The listing builds one solid part. Answer for the finished solid, in the listing's coordinates (mm). Face numbers are marked on the shaded views. A direction names the side the tool comes from. Coordinates: 2 decimals unless noted, no trailing zeros. Write each loop counter-clockwise with the first axis right and the second up, starting at its lowest first coordinate (ties: lowest second). Pieces come first, ordered by that corner, then holes.
(1) The part is cut by section A-A on z = 0. Determine the outline of the cut face in (x, y), plus the area to 3 significant figures.
(2) Given P1, Ø1.5, axis at y = 50.5, z = -0.5, coming from the +X side; P2, Ø18, axis at x = 49, z = -6.5, coming from the +Y side, each flat-ended and moving along its own axis, determine where each tip first touches the part or whether it passes through.
(3) Which of the six approach directions +Z, -Z, +X, -X, +Y, -Y give full straight-line access (tool end or side, diameter ignored) to the marked faces 1 and 2?
(4) The part is cut by section B-B on y = 60. Determine the outline of the cut face in (x, z), plus the area to 3 significant figures.
(5) The part is cut by section D-D on z = -5.5. Determine the outline of the cut face in (x, y).
(6) Straight lines are drawn through the part: line 1 (Z direction, x = 4, y = 20); line 2 (Y direction, x = 3.8, z = 0); line 3 (Y direction, x = 4.55, z = 0). For each, find the intervals that lie inside material, in ascending order.
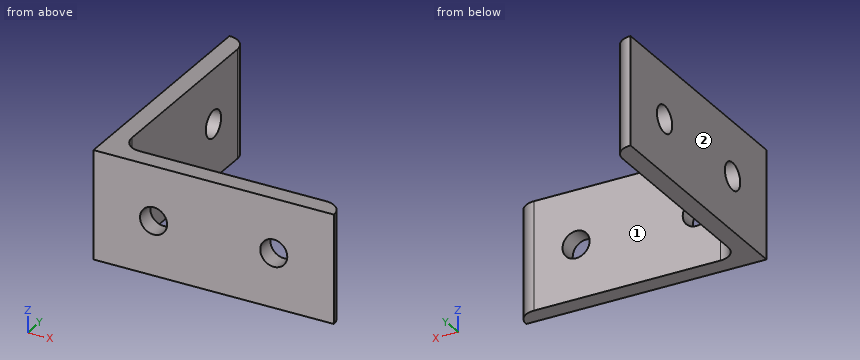
from build123d import *

# Parameters (mm, degrees)
BOSS_EXTRUDE1_DEPTH = 18
SKETCH2_R           = 4.5
CUT_EXTRUDE1_DEPTH  = 81
SKETCH3_R           = 4.5
CUT_EXTRUDE2_DEPTH  = 81


with BuildPart() as part:
    # Sketch1 → Boss-Extrude1 (new body, symmetric)
    with BuildSketch(Plane.XY):
        with BuildLine():
            Line((0, 0), (0, 80))
            ThreePointArc((0, 80), (4.242640687, 78.242640687), (6, 74))
            Line((6, 74), (6, 12))
            ThreePointArc((6, 12), (7.757359313, 7.757359313), (12, 6))
            Line((12, 6), (74, 6))
            ThreePointArc((74, 6), (78.242640687, 4.242640687), (80, 0))
            Line((80, 0), (0, 0))
        make_face()
    extrude(amount=BOSS_EXTRUDE1_DEPTH, both=True)

    # Sketch2 → Cut-Extrude1 (cut, through all)
    with BuildSketch(Plane(origin=(0, 0, 0), x_dir=(1, 0, 0), z_dir=(0, 1, 0))):
        with Locations((20, 0)):
            Circle(SKETCH2_R)
        with Locations((60, 0)):
            Circle(SKETCH2_R)
    extrude(amount=CUT_EXTRUDE1_DEPTH, mode=Mode.SUBTRACT)

    # Sketch3 → Cut-Extrude2 (cut, through all)
    with BuildSketch(Plane(origin=(0, 0, 0), x_dir=(0, 0, -1), z_dir=(1, 0, 0))):
        with Locations((0, 20)):
            Circle(SKETCH3_R)
        with Locations((0, 60)):
            Circle(SKETCH3_R)
    extrude(amount=CUT_EXTRUDE2_DEPTH, mode=Mode.SUBTRACT)


solid = part.part
Model answer:
1. outline: (0, 0) - (15.5, 0) - (15.5, 6) - (12, 6) arc R6 cw to (6, 12) - (6, 15.5) - (0, 15.5) - close; (0, 24.5) - (6, 24.5) - (6, 55.5) - (0, 55.5) - close; (0, 64.5) - (6, 64.5) - (6, 74) arc R6 ccw to (0, 80) - close; (24.5, 0) - (55.5, 0) - (55.5, 6) - (24.5, 6) - close; (64.5, 0) - (80, 0) arc R6 ccw to (74, 6) - (64.5, 6) - close
1. area: 700 mm2
2. P1: stops at x = 6
2. P2: stops at y = 6
3. face 1: +Z, -Z, +X, +Y
3. face 2: +Z, -Z, -X, +Y, -Y
4. outline: (0, -18) - (6, -18) - (6, -4.5) - (0, -4.5) - close; (0, 4.5) - (6, 4.5) - (6, 18) - (0, 18) - close
4. area: 162 mm2
5. outline: (0, 0) - (80, 0) arc R6 ccw to (74, 6) - (12, 6) arc R6 cw to (6, 12) - (6, 74) arc R6 ccw to (0, 80) - close
6. line 1: z = -18 to -4.5, 4.5 to 18
6. line 2: y = 0 to 15.5, 24.5 to 55.5, 64.5 to 78.64
6. line 3: y = 0 to 15.5, 24.5 to 55.5, 64.5 to 77.91
